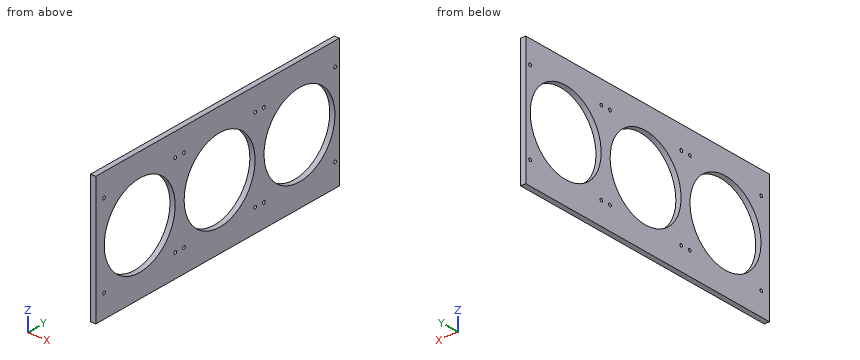
```python
from build123d import *

# Parameters (mm, degrees)
SKETCH1_W                     = 166.5
SKETCH1_H                     = 111
BOSS_EXTRUDE1_DEPTH           = 30.5
SHELL1_T                      = -4.5
CUT_EXTRUDE1_REACH            = 105.377
SKETCH2_W                     = 157
SKETCH2_H                     = 92
TAP_DRILL_FOR_6_32_TAP1_D     = 2.7051
TAP_DRILL_FOR_6_32_TAP1_DEPTH = 4.5
LPATTERN1_COUNT               = 8
LPATTERN1_PITCH               = 30.5
SKETCH7_W                     = 102
SKETCH7_H                     = 4.5
CUT_EXTRUDE2_DEPTH            = 5
SKETCH8_W                     = 102
SKETCH8_H                     = 157
CUT_EXTRUDE3_DEPTH            = 5
CUT_EXTRUDE4_REACH            = 302.564
SKETCH9_R                     = 35.5
TAP_DRILL_FOR_6_32_TAP2_D     = 2.7051
CUT_EXTRUDE6_START            = -162
SKETCH14_W                    = 111
SKETCH14_H                    = 244
CUT_EXTRUDE6_DEPTH            = 162


with BuildPart() as part:
    # Sketch1 → Boss-Extrude1 (new body)
    with BuildSketch(Plane(origin=(0, 0, 0), x_dir=(1, 0, 0), z_dir=(0, 1, 0))):
        Rectangle(SKETCH1_W, SKETCH1_H)
    extrude(amount=BOSS_EXTRUDE1_DEPTH)

    # Shell1
    shell1_openings = [part.faces().sort_by_distance(p)[0] for p in [
        (0, 30.5, 0),
        (-83.25, 15.25, 0),
    ]]
    offset(amount=SHELL1_T, openings=shell1_openings, kind=Kind.INTERSECTION)

    # Sketch2 → Cut-Extrude1 (cut, up to next)
    with BuildSketch(Plane(origin=(0, 4.5, 0), x_dir=(1, 0, 0), z_dir=(0, 1, 0)), mode=Mode.PRIVATE) as cut_extrude1_sk1:
        with Locations((0.25, 0)):
            Rectangle(SKETCH2_W, SKETCH2_H)
    cut_extrude1_tool1 = extrude(cut_extrude1_sk1.sketch, amount=-CUT_EXTRUDE1_REACH, mode=Mode.PRIVATE) & part.part
    add(cut_extrude1_tool1.solids().sort_by_distance((0.25, 4.5, 0))[0], mode=Mode.SUBTRACT)

    # Tap Drill for #6-32 Tap1
    with Locations(Plane(origin=(0, 0, -55.5), x_dir=(-1, 0, 0), z_dir=(0, 0, -1))):
        with Locations((42.66, 10.84), (-58.75, 10.84)):
            tap_drill_for_6_32_tap1 = Hole(TAP_DRILL_FOR_6_32_TAP1_D / 2, depth=TAP_DRILL_FOR_6_32_TAP1_DEPTH)

    # Mirror1: Tap Drill for #6-32 Tap1 across plane
    add(tap_drill_for_6_32_tap1.mirror(Plane.XY), mode=Mode.SUBTRACT)


with BuildPart() as lpattern1_1:
    # LPattern1: pattern copy
    add(part.part.moved(Location(Vector(0, 1, 0) * (1 * LPATTERN1_PITCH))))


with BuildPart() as lpattern1_2:
    # LPattern1: pattern copy
    add(part.part.moved(Location(Vector(0, 1, 0) * (2 * LPATTERN1_PITCH))))


with BuildPart() as lpattern1_3:
    # LPattern1: pattern copy
    add(part.part.moved(Location(Vector(0, 1, 0) * (3 * LPATTERN1_PITCH))))


with BuildPart() as lpattern1_4:
    # LPattern1: pattern copy
    add(part.part.moved(Location(Vector(0, 1, 0) * (4 * LPATTERN1_PITCH))))


with BuildPart() as lpattern1_5:
    # LPattern1: pattern copy
    add(part.part.moved(Location(Vector(0, 1, 0) * (5 * LPATTERN1_PITCH))))


with BuildPart() as lpattern1_6:
    # LPattern1: pattern copy
    add(part.part.moved(Location(Vector(0, 1, 0) * (6 * LPATTERN1_PITCH))))


with BuildPart() as lpattern1_7:
    # LPattern1: pattern copy
    add(part.part.moved(Location(Vector(0, 1, 0) * (7 * LPATTERN1_PITCH))))


with BuildPart() as part_1:
    add(part.part)

    # Combine1: union LPattern1_1
    add(lpattern1_1.part)

    # Sketch7 → Cut-Extrude2 (cut)
    with BuildSketch(Plane.ZY.offset(83.25)):
        with Locations((0, 32.75)):
            Rectangle(SKETCH7_W, SKETCH7_H)
    extrude(amount=-CUT_EXTRUDE2_DEPTH, mode=Mode.SUBTRACT)


with BuildPart() as lpattern1_2_1:
    add(lpattern1_2.part)

    # Combine2: union LPattern1_3, LPattern1_5, LPattern1_4, LPattern1_7, part, LPattern1_6
    add(lpattern1_3.part)
    add(lpattern1_5.part)
    add(lpattern1_4.part)
    add(lpattern1_7.part)
    add(part_1.part)
    add(lpattern1_6.part)

    # Sketch8 → Cut-Extrude3 (cut)
    with BuildSketch(Plane.ZY.offset(83.25)):
        with Locations((0, 139.5)):
            Rectangle(SKETCH8_W, SKETCH8_H)
    extrude(amount=-CUT_EXTRUDE3_DEPTH, mode=Mode.SUBTRACT)

    # Sketch9 → Cut-Extrude4 (cut, up to next)
    with BuildSketch(Plane(origin=(83.25, 0, 0), x_dir=(0, 0, -1), z_dir=(1, 0, 0)), mode=Mode.PRIVATE) as cut_extrude4_sk1:
        with Locations((0, 204)):
            Circle(SKETCH9_R)
    cut_extrude4_tool1 = extrude(cut_extrude4_sk1.sketch, amount=-CUT_EXTRUDE4_REACH, mode=Mode.PRIVATE) & lpattern1_2_1.part
    # Sketch9 → Cut-Extrude4 (cut, up to next)
    with BuildSketch(Plane(origin=(83.25, 0, 0), x_dir=(0, 0, -1), z_dir=(1, 0, 0)), mode=Mode.PRIVATE) as cut_extrude4_sk2:
        with Locations((0, 124)):
            Circle(SKETCH9_R)
    cut_extrude4_tool2 = extrude(cut_extrude4_sk2.sketch, amount=-CUT_EXTRUDE4_REACH, mode=Mode.PRIVATE) & lpattern1_2_1.part
    # Sketch9 → Cut-Extrude4 (cut, up to next)
    with BuildSketch(Plane(origin=(83.25, 0, 0), x_dir=(0, 0, -1), z_dir=(1, 0, 0)), mode=Mode.PRIVATE) as cut_extrude4_sk3:
        with Locations((0, 44)):
            Circle(SKETCH9_R)
    cut_extrude4_tool3 = extrude(cut_extrude4_sk3.sketch, amount=-CUT_EXTRUDE4_REACH, mode=Mode.PRIVATE) & lpattern1_2_1.part
    add(cut_extrude4_tool1.solids().sort_by_distance((83.25, 204, 0))[0], mode=Mode.SUBTRACT)
    add(cut_extrude4_tool2.solids().sort_by_distance((83.25, 124, 0))[0], mode=Mode.SUBTRACT)
    add(cut_extrude4_tool3.solids().sort_by_distance((83.25, 44, 0))[0], mode=Mode.SUBTRACT)

    # Tap Drill for #6-32 Tap2 (through all)
    with Locations(Plane(origin=(83.25, 0, 0), x_dir=(0, 0, -1), z_dir=(1, 0, 0))):
        with Locations((-35.675, 239.675), (35.675, 239.675), (35.675, 168.325), (-35.675, 168.325)):
            tap_drill_for_6_32_tap2 = Hole(TAP_DRILL_FOR_6_32_TAP2_D / 2)

    # Mirror2: Tap Drill for #6-32 Tap2 across plane
    add(tap_drill_for_6_32_tap2.mirror(Plane.ZX.offset(164)), mode=Mode.SUBTRACT)

    # Mirror3: Tap Drill for #6-32 Tap2 across plane
    add(tap_drill_for_6_32_tap2.mirror(Plane.ZX.offset(124)), mode=Mode.SUBTRACT)

    # Sketch14 → Cut-Extrude6 (cut)
    with BuildSketch(Plane.ZY.offset(83.25).offset(CUT_EXTRUDE6_START)):
        with Locations((0, 122)):
            Rectangle(SKETCH14_W, SKETCH14_H)
    extrude(amount=CUT_EXTRUDE6_DEPTH, mode=Mode.SUBTRACT)


solid = lpattern1_2_1.part
```
CAD build for the part. Positions are in the model's coordinates, mm. Coordinates: 2 decimals unless noted, no trailing zeros. Loops run counter-clockwise (first coordinate to the right, second up) from the corner with the lowest first, then second, coordinate; pieces in that order, holes last. Notation, with made-up numbers: (-14.75, 62) - (2.25, 62) arc R27 ccw to (2.25, 98) - close; hole circle Ø1 at (32.25, 60.5). An arc over 180 degrees is marked (long way). Use CSV: the item, a comma, the result in double quotes. Start each with the question number.
Q1. Probe probe 1 along Y at (x, z) = (82, 0); probe 2 along Y at (x, z) = (82.4, 8); probe 3 along Z at (x, y) = (82.4, 199.5). List the from-to ranges inside material, lowest first. Write a range as from..to.
Q2. Cut at D-D, the plane y = 188. List the corners of the cut face in (x, z).
Q3. Cut at C-C, the plane z = 16. List the corners of the cut face in (x, y).
Q4. Cut at B-B, the plane x = 79.65. State how many separate pieces and enclosed holes the cut face has, then the cut area to 3 significant figures.
Q5. Cut at A-A, the plane y = 44. List the corners of the cut face in (x, z), then the cut area to 3 significant figures.
Here are the results:
1,probe 1,"0..8.5, 79.5..88.5, 159.5..168.5, 239.5..244"
1,probe 2,"0..9.41, 78.59..89.41, 158.59..169.41, 238.59..244"
1,probe 3,"-55.5..-35.21, 35.21..55.5"
2,outline,"(78.75, -55.5) - (83.25, -55.5) - (83.25, -31.69) - (78.75, -31.69) - close; (78.75, 31.69) - (83.25, 31.69) - (83.25, 55.5) - (78.75, 55.5) - close"
3,outline,"(78.75, 0) - (83.25, 0) - (83.25, 12.31) - (78.75, 12.31) - close; (78.75, 75.69) - (83.25, 75.69) - (83.25, 92.31) - (78.75, 92.31) - close; (78.75, 155.69) - (83.25, 155.69) - (83.25, 172.31) - (78.75, 172.31) - close; (78.75, 235.69) - (83.25, 235.69) - (83.25, 244) - (78.75, 244) - close"
4,separate pieces,"1"
4,enclosed holes,"15"
4,area,"15,100 mm2"
5,outline,"(78.75, -55.5) - (83.25, -55.5) - (83.25, -35.5) - (78.75, -35.5) - close; (78.75, 35.5) - (83.25, 35.5) - (83.25, 55.5) - (78.75, 55.5) - close"
5,area,"180 mm2"
